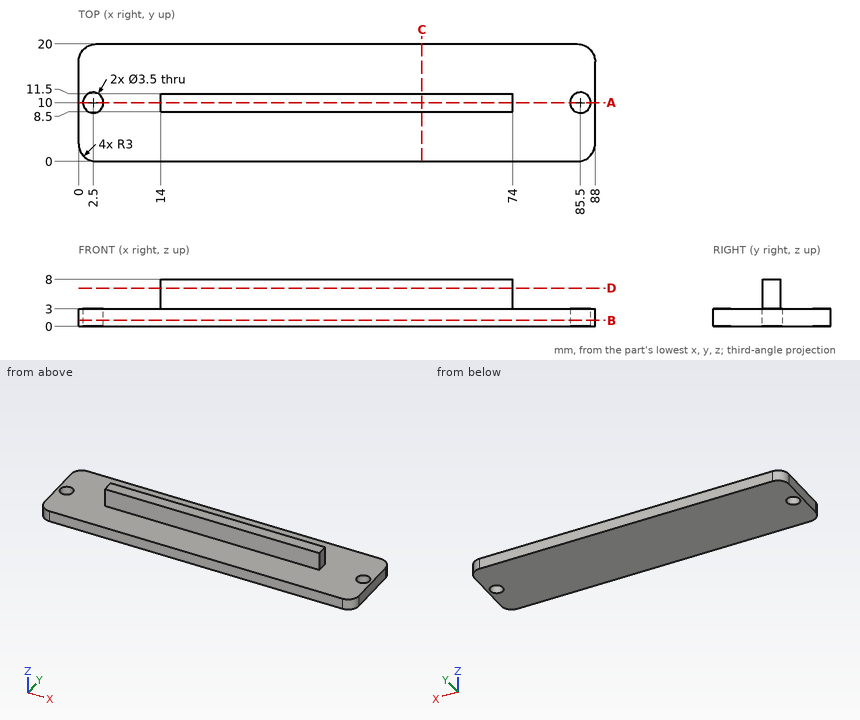
For this review, use the dimensioned drawing (mm, ordinates from the lowest corner) and the shaded views. Round coordinates to 2 decimals unless told otherwise and drop trailing zeros. Write each loop counter-clockwise with the first axis right and the second up, starting at its lowest first coordinate (ties: lowest second). Pieces come first, ordered by that corner, then holes. Notation, with made-up numbers: M -16.5,32 L 34.5,32 A24 cw 34.5,68 Z; hole C -22,29.25 d1. An arc over 180 degrees is marked long. Write item = value, one per line. Start each with the question number.
(1) For line 1 along Z through (x, y) = (73, 5.5); line 2 along Y through (x, z) = (2.5, 1.6); line 3 along Y through (x, z) = (49.5, 5.75), list the stretches that pass through material, from the lowest coordinate up.
(2) We need section B-B (z = 1). Give the boundary of the cut face in (x, y).
(3) We need section A-A (y = 10). Give the boundary of the cut face in (x, z), then the cut area to 3 significant figures.
(4) We need section D-D (z = 6.5). Give the boundary of the cut face in (x, y).
(5) We need section C-C (x = 58.5). Give the boundary of the cut face in (y, z).
(6) Clearance check with flat-ended pins moving along their axes: pin 1 Ø3.5 at (y, z) = (9.5, 5) entering from -X; pin 2 Ø2.5 at (y, z) = (10.5, 4.5) entering from +X; pin 3 Ø3 at (x, z) = (23.5, 7) entering from +Y; pin 4 Ø3 at (x, y) = (2.5, 10) entering from -Z. State where each tip first meets the part, or that it passes through.
Results found:
q1.line_1 = 0 to 3
q1.line_2 = 0.04 to 8.25, 11.75 to 19.96
q1.line_3 = 8.5 to 11.5
q2.outline = M 0,3 A3 ccw 3,0 L 85,0 A3 ccw 88,3 L 88,17 A3 ccw 85,20 L 3,20 A3 ccw 0,17 Z; hole C 2.5,10 d3.5; hole C 85.5,10 d3.5
q3.outline = M 0,0 L 0.75,0 L 0.75,3 L 0,3 Z; M 4.25,0 L 83.75,0 L 83.75,3 L 74,3 L 74,8 L 14,8 L 14,3 L 4.25,3 Z; M 87.25,0 L 88,0 L 88,3 L 87.25,3 Z
q3.area = 543 mm²
q4.outline = M 14,8.5 L 74,8.5 L 74,11.5 L 14,11.5 Z
q5.outline = M 0,0 L 20,0 L 20,3 L 11.5,3 L 11.5,8 L 8.5,8 L 8.5,3 L 0,3 Z
q6.pin_1 = 14
q6.pin_2 = 74
q6.pin_3 = 11.5
q6.pin_4 = through
